Source: CAD feature listing. Evaluate the final solid. Frame: model axes, mm. A direction names the side the tool comes from. Round coordinates to 2 decimals unless told otherwise and drop trailing zeros. Loops run counter-clockwise (first coordinate to the right, second up) from the corner with the lowest first, then second, coordinate; pieces in that order, holes last. Notation, with made-up numbers: M -22.5,-15 L 25.5,-15 A22 ccw 25.5,1 Z; hole C 85,27 d4. An arc over 180 degrees is marked long. Answer as CSV lines item,"result". Start each with the question number.
```python
from build123d import *

# Parameters (mm, degrees)
F0_W     = 384.636849165
F0_H     = 264.3615156412
F1_DEPTH = 322.58
F2_W     = 384.636849165
F2_H     = 129.9396157265
F3_DEPTH = 135.636
F4_DEPTH = 158.75
F5_T     = -2.54
F6_W     = 140.2605473995
F6_H     = 39.0601313553
F7_DEPTH = 25.4
F8_R     = 21.6824210641
F9_DEPTH = 25.4


with BuildPart() as f1:
    # F0 (on Top) → F1 (new body)
    with BuildSketch(Plane.XY):
        with Locations((9.9443048239, 2.2411420941)):
            Rectangle(F0_W, F0_H)
    extrude(amount=F1_DEPTH)

    # F2 (on face) → F3 (cut)
    with BuildSketch(Plane.XY.offset(322.58)):
        with Locations((9.9443048239, -64.9698078632)):
            Rectangle(F2_W, F2_H)
    extrude(amount=-F3_DEPTH, mode=Mode.SUBTRACT)

    # F4 (add): a face of the model
    f4_faces = [f1.faces().sort_by_distance(p)[0] for p in [
        (9.9443048239, 134.4218999147, 161.29),
    ]]
    extrude(f4_faces, amount=F4_DEPTH)

    # F5
    f5_openings = [f1.faces().sort_by_distance(p)[0] for p in [
        (9.944305, 293.1719, 161.29),
    ]]
    offset(amount=F5_T, openings=f5_openings, kind=Kind.INTERSECTION)

    # F6 (on face) → F7 (cut)
    with BuildSketch(Plane(origin=(0, 2.54, 0), x_dir=(-1, 0, 0), z_dir=(0, 1, 0))):
        with Locations((-0.2779662609, 203.9340656776)):
            Rectangle(F6_W, F6_H)
    extrude(amount=-F7_DEPTH, mode=Mode.SUBTRACT)

    # F8 (on face) → F9 (cut)
    with BuildSketch(Plane.XZ):
        with Locations((0, 273.7638354301)):
            Circle(F8_R)
    extrude(amount=-F9_DEPTH, mode=Mode.SUBTRACT)


solid = f1.part
```
1) Section B-B, the plane y = -47.5. Return loops of the section in (x, z), and give its area (3 significant figures).
2) Contact query for flat-ended pins moving along their axis: pin 1 Ø6 at (x, z) = (-52, 254) entering from +Y; pin 2 Ø1.3 at (x, z) = (-10.5, 186) entering from +Y; pin 3 Ø12 at (x, z) = (8.5, 46) entering from +Y. Output: stop coordinate, or through.
3) Access query for faces 1 (the flat face through (7, 2.54, 253)), 2 (the flat face through (7, 145, 322.58)), 3 (the flat face through (7, -64, 186.944)). Directions: +Z, -Z, +X, -X, +Y, -Y. A direction counts if a zero-diameter tool reaches every point of the face in a straight line with its end or side. Return the directions, or none.
4) Mould query, pull axis X, two halves, no side actions, for faces 4 (the flat face through (-182.374, 126, 159)), 5 (the flat face through (7, 79, 0)), 6 (the flat face through (202.263, 126, 159)), 7 (the flat face through (-69.852, 0.2, 195.2)). Classes: pulls with the +X half, pulls with the -X half, needs draft (parallel to the pull), parting line crosses it, or undercut.
5) Ray query, line 1 along Z through (x, y) = (0, 0.65); line 2 along X through (y, z) = (15, 28); line 3 along Z through (x, y) = (56, 179). Return the intervals inside material, ascending.
6) Section D-D, the plane z = 111.5. Return loops of the section in (x, y), and give its area (3 significant figures).
7) Section C-C, the plane x = 51. Return loops of the section in (y, z).
8) Section A-A, the plane x = 0. Return loops of the section in (y, z).
Findings below:
1,outline,"M -182.37,0 L 202.26,0 L 202.26,186.94 L -182.37,186.94 Z; hole M -179.83,2.54 L 199.72,2.54 L 199.72,184.4 L -179.83,184.4 Z"
1,area,"2,880 mm²"
2,pin 1,"y = 2.54"
2,pin 2,"y = -22.86"
2,pin 3,"y = -127.4"
3,face 1,"+Y"
3,face 2,"+Z, +X, -X, +Y, -Y"
3,face 3,"+Z, +X, -X, -Y"
4,face 4,"pulls with the -X half"
4,face 5,"needs draft"
4,face 6,"pulls with the +X half"
4,face 7,"undercut"
5,line 1,"0 to 2.54, 223.46 to 252.08, 295.45 to 322.58"
5,line 2,"-182.37 to -179.83, 199.72 to 202.26"
5,line 3,"0 to 2.54, 320.04 to 322.58"
6,outline,"M -182.37,-129.94 L 202.26,-129.94 L 202.26,293.17 L 199.72,293.17 L 199.72,-127.4 L -179.83,-127.4 L -179.83,293.17 L -182.37,293.17 Z"
6,area,"3,110 mm²"
7,outline,"M -129.94,0 L 293.17,0 L 293.17,2.54 L -127.4,2.54 L -127.4,184.4 L -22.86,184.4 L -22.86,186.94 L -129.94,186.94 Z; M 0,223.46 L 2.54,223.46 L 2.54,320.04 L 293.17,320.04 L 293.17,322.58 L 0,322.58 Z"
8,outline,"M -129.94,0 L 293.17,0 L 293.17,2.54 L -127.4,2.54 L -127.4,184.4 L -22.86,184.4 L -22.86,186.94 L -129.94,186.94 Z; M 0,223.46 L 2.54,223.46 L 2.54,252.08 L 0,252.08 Z; M 0,295.45 L 2.54,295.45 L 2.54,320.04 L 293.17,320.04 L 293.17,322.58 L 0,322.58 Z"
